from build123d import *

# Parameters (mm, degrees)
SKETCH_1_W               = 110
SKETCH_1_H               = 155
EXTRUDE_1_DEPTH          = 10
CUT_EXTRUDE_1_DEPTH      = 96.557574268
CUT_EXTRUDE_1_DEPTH_BACK = 96.557574268


with BuildPart() as part:
    # 草图1 → 凸台-拉伸1 (new body)
    with BuildSketch(Plane.XY):
        Rectangle(SKETCH_1_W, SKETCH_1_H)
    extrude(amount=EXTRUDE_1_DEPTH)

    # 草图2 → 切除-拉伸1 (cut, two sides: drawn at the far end of the back side and taken through both)
    with BuildSketch(Plane.XY.offset(10).offset(-CUT_EXTRUDE_1_DEPTH_BACK)):
        with BuildLine():
            Line((-27.75, -24.25), (-7.75, -24.25))
            ThreePointArc((-7.75, -24.25), (0.25, -32.25), (-7.75, -40.25))
            Line((-7.75, -40.25), (-27.75, -40.25))
            ThreePointArc((-27.75, -40.25), (-35.75, -32.25), (-27.75, -24.25))
        make_face()
    extrude(amount=CUT_EXTRUDE_1_DEPTH + CUT_EXTRUDE_1_DEPTH_BACK, mode=Mode.SUBTRACT)


solid = part.part
Here's how the part is built. I have some questions about the finished solid (model axes, mm). A direction names the side the tool comes from. Coordinates: 2 decimals unless noted, no trailing zeros. Order: outer loops, then holes, each group sorted by start corner. A loop starts at its lowest first (then second) coordinate and runs counter-clockwise, first axis right, second up.
Item 1: If we section it at C-C on z = 5.25: List the corners of the cut face in (x, y) for me, plus the area to 3 significant figures.
Result sheet:
outline: (-55, -77.5) - (55, -77.5) - (55, 77.5) - (-55, 77.5) - close; hole (-27.75, -40.25) - (-7.75, -40.25) arc R8 ccw to (-7.75, -24.25) - (-27.75, -24.25) arc R8 ccw to start
area: 16,500 mm2
Item 2: If we section it at A-A on x = -23.5: List the corners of the cut face in (y, z) for me, plus the area to 3 significant figures.
Result sheet:
outline: (-77.5, 0) - (-40.25, 0) - (-40.25, 10) - (-77.5, 10) - close; (-24.25, 0) - (77.5, 0) - (77.5, 10) - (-24.25, 10) - close
area: 1,390 mm2
Item 3: If we section it at B-B on y = -32.25: List the corners of the cut face in (x, z) for me.
Result sheet:
outline: (-55, 0) - (-35.75, 0) - (-35.75, 10) - (-55, 10) - close; (0.25, 0) - (55, 0) - (55, 10) - (0.25, 10) - close
Item 4: If we mould it in two halves opening along X, with no side actions, what happens to faces 3 (the face through (-18, -24.25, 5)), 4 (the face through (-1, -77.5, 5)), 5 (the face through (-18, -40.25, 5)), 6 (the face through (-55, -1, 5))? For each: +X half, -X half, draft (parallel to the pull), parting line (faces both ways), or undercut.
Result sheet:
face 3: undercut
face 4: draft
face 5: undercut
face 6: -X half
Item 5: I need wall thicknesses on line 1 (Y direction, x = -8, z = 4.5); line 2 (X direction, y = -34, z = 1.5). Which ranges of each line are inside material? Lowest first, please.
Result sheet:
line 1: y = -77.5 to -40.25, -24.25 to 77.5
line 2: x = -55 to -35.56, 0.06 to 55
Item 6: For faces 1 (the face through (0.248, -32.074, 4.93)), 2 (the face through (-1, 77.5, 5)), which set-ups out of +Z, -Z, +X, -X, +Y, -Y let a thin tool reach every point of the face, with its end or its side?
Result sheet:
face 1: +Z, -Z
face 2: +Z, -Z, +X, -X, +Y
